Build history of the part. All positions in model axes, mm. A direction names the side the tool comes from. Round coordinates to 2 decimals unless told otherwise and drop trailing zeros. Order: outer loops, then holes, each group sorted by start corner. A loop starts at its lowest first (then second) coordinate and runs counter-clockwise, first axis right, second up. Notation, with made-up numbers: M 27,63 L 64,63 A27 cw 64,98 Z; hole C -22.5,-4 d1. An arc over 180 degrees is marked long. One line per item, written item: value. Start each with the question number.
Item 1: Band-saw the part on A-A, the plane z = -50.8. Write the cut outline in (x, y) (3 decimals).
Item 2: Two-plate mould, pull along Z, no slides. Class faces 4 (the flat face through (8.179, 2, -9)), 5 (the flat face through (50.8, 2, -70)), 6 (the cylindrical face through (11.936, 1.61, -0.724)): +Z half, -Z half, draft (parallel to the pull), parting line (faces both ways), or undercut.
Item 3: Band-saw the part on C-C, the plane y = 2.6. Write the cut outline in (x, z) (3 decimals).
Item 4: Tool access for faces 1 (the flat face through (33, 2, -63.5)), 2 (the flat face through (8.179, 2, -47)), 3 (the cylindrical face through (0.724, 1.61, -75.436)): list every direction of +Z, -Z, +X, -X, +Y, -Y with a clear straight run to the whole face (end or side of a thin tool).
Item 5: Probe L1, parallel to X at y = 2.5, z = -69.85 (3 decimals); L2, parallel to X at y = 0.7, z = -12.7 (3 decimals); L3, parallel to X at y = 1.8, z = -27.5. List the from-to ranges inside material, lowest first.
Item 6: Pin check, flat tips, straight feed: pin 1 (5.5 mm diameter, centred on x = 6.35, z = -12.7, fed in from +Y); pin 2 (1 mm diameter, centred on y = 1, z = -24, fed in from +X); pin 3 (1.6 mm diameter, centred on x = 40, y = 1, fed in from +Z). Stop position of each tip, or through.
Item 7: Band-saw the part on B-B, the plane x = 31.75. Write the cut outline in (y, z) (3 decimals).
Item 8: Band-saw the part on D-D, the plane x = 6.35. Write the cut outline in (y, z) (3 decimals), then the cut area to 3 significant figures.
```python
from build123d import *

# Parameters (mm, degrees)
BOSS_EXTRUDE1_DEPTH = 3.175
SKETCH2_R           = 1.905
CUT_EXTRUDE1_DEPTH  = 3.175
FILLET3_R           = 2.54


with BuildPart() as part:
    # Sketch1 → Boss-Extrude1 (new body)
    with BuildSketch(Plane(origin=(0, 0, 0), x_dir=(1, 0, 0), z_dir=(0, 1, 0))):
        Polygon((0, 76.2), (0, 0), (12.7, 0), (12.7, 63.5), (50.8, 63.5), (50.8, 76.2), align=None)
    extrude(amount=BOSS_EXTRUDE1_DEPTH)

    # Sketch2 → Cut-Extrude1 (cut)
    with BuildSketch(Plane(origin=(0, 3.175, 0), x_dir=(1, 0, 0), z_dir=(0, 1, 0))):
        with BuildLine():
            Line((4.5212, 48.204597226), (4.5212, 45.72))
            ThreePointArc((4.5212, 45.72), (6.35, 43.8912), (8.1788, 45.72))
            Line((8.1788, 45.72), (8.1788, 48.204597226))
            ThreePointArc((8.1788, 48.204597226), (6.35, 53.975), (4.5212, 48.204597226))
        make_face()
        with BuildLine():
            Line((4.5212, 10.104597226), (4.5212, 7.62))
            ThreePointArc((4.5212, 7.62), (6.35, 5.7912), (8.1788, 7.62))
            Line((8.1788, 7.62), (8.1788, 10.104597226))
            ThreePointArc((8.1788, 10.104597226), (6.35, 15.875), (4.5212, 10.104597226))
        make_face()
        with Locations(Location((31.75, 69.85, 0), (0, 0, 270))):
            Circle(SKETCH2_R)
        with Locations(Location((6.35, 69.85, 0), (0, 0, 270))):
            Circle(SKETCH2_R)
    extrude(amount=-CUT_EXTRUDE1_DEPTH, mode=Mode.SUBTRACT)

    # Fillet3
    fillet3_edges = [part.edges().sort_by_distance(p)[0] for p in [
        (12.7, 1.5875, -63.5),
        (12.7, 1.5875, 0),
        (0, 1.5875, 0),
        (0, 1.5875, -76.2),
    ]]
    fillet(fillet3_edges, radius=FILLET3_R)


solid = part.part
```
Output:
1. outline: M 0,0 L 3.175,0 L 3.175,3.175 L 0,3.175 Z; M 9.525,0 L 12.7,0 L 12.7,3.175 L 9.525,3.175 Z
2. face 4: undercut
2. face 5: draft
2. face 6: +Z half
3. outline: M 0,-73.66 A2.54 ccw 2.54,-76.2 L 50.8,-76.2 L 50.8,-63.5 L 15.24,-63.5 A2.54 cw 12.7,-60.96 L 12.7,-2.54 A2.54 ccw 10.16,0 L 2.54,0 A2.54 ccw 0,-2.54 Z; hole C 6.35,-69.85 d3.81; hole M 4.521,-48.205 A3.175 ccw long 8.179,-48.205 L 8.179,-45.72 A1.829 ccw 4.521,-45.72 Z; hole M 4.521,-10.105 A3.175 ccw long 8.179,-10.105 L 8.179,-7.62 A1.829 ccw 4.521,-7.62 Z; hole C 31.75,-69.85 d3.81
4. face 1: +Z, +X, +Y, -Y
4. face 2: +Y, -Y
4. face 3: -Z, -X, +Y, -Y
5. L1: x = 0 to 4.445, 8.255 to 29.845, 33.655 to 50.8
5. L2: x = 0 to 3.175, 9.525 to 12.7
5. L3: x = 0 to 12.7
6. pin 1: passes through
6. pin 2: stops at x = 12.7
6. pin 3: stops at z = -63.5
7. outline: M 0,-76.2 L 3.175,-76.2 L 3.175,-71.755 L 0,-71.755 Z; M 0,-67.945 L 3.175,-67.945 L 3.175,-63.5 L 0,-63.5 Z
8. outline: M 0,-76.2 L 3.175,-76.2 L 3.175,-71.755 L 0,-71.755 Z; M 0,-67.945 L 3.175,-67.945 L 3.175,-53.975 L 0,-53.975 Z; M 0,-43.891 L 3.175,-43.891 L 3.175,-15.875 L 0,-15.875 Z; M 0,-5.791 L 3.175,-5.791 L 3.175,0 L 0,0 Z
8. area: 166 mm²
